from build123d import *

# Parameters (mm, degrees)
SKETCH1_R           = 3.1877
BOSS_EXTRUDE1_DEPTH = 9.525


with BuildPart() as part:
    # Sketch1 → Boss-Extrude1 (new body)
    with BuildSketch(Plane.XY):
        with BuildLine():
            Line((-19.84375, -1.016), (-18.881836189, -1.016))
            ThreePointArc((-18.881836189, -1.016), (-13.4874, 1.4478), (-8.092963811, -1.016))
            Line((-8.092963811, -1.016), (12.583078625, -6.944759764))
            ThreePointArc((12.583078625, -6.944759764), (19.827318682, -1.116916975), (13.49375, 5.6896))
            Line((13.49375, 5.6896), (-13.49375, 5.6896))
            ThreePointArc((-13.49375, 5.6896), (-17.983878061, 3.829728061), (-19.84375, -0.6604))
            Line((-19.84375, -0.6604), (-19.84375, -1.016))
        make_face()
        with Locations((13.49375, -0.6604)):
            Circle(SKETCH1_R, mode=Mode.SUBTRACT)
    extrude(amount=-BOSS_EXTRUDE1_DEPTH)


solid = part.part
The listing builds one solid part. Answer for the finished solid, in the listing's coordinates (mm). A direction names the side the tool comes from. Give positions to 0.01 mm unless a question says otherwise; leave off trailing zeros. Order: outer loops, then holes, each group sorted by start corner. A loop starts at its lowest first (then second) coordinate and runs counter-clockwise, first axis right, second up. Notation, with made-up numbers: (9, 71.25) - (21, 71.25) arc R12 cw to (21, 90.25) - close; hole circle Ø10 at (-38.5, 34). An arc over 180 degrees is marked (long way). Use one line per item in the form item = value.
1) Find section B-B on z = -7.75. Determine the outline of the cut face in (x, y), and give its area (3 significant figures).
Verdict:
outline = (-19.84, -1.02) - (-18.88, -1.02) arc R7.14 cw to (-8.09, -1.02) - (12.58, -6.94) arc R6.35 ccw (long way) to (13.49, 5.69) - (-13.49, 5.69) arc R6.35 ccw to (-19.84, -0.66) - close; hole circle Ø6.38 at (13.49, -0.66)
area = 295 mm^2
2) Find section C-C on x = 15.5. Determine the outline of the cut face in (y, z) (3 decimals).
Verdict:
outline = (-6.685, -9.525) - (-3.138, -9.525) - (-3.138, 0) - (-6.685, 0) - close; (1.817, -9.525) - (5.364, -9.525) - (5.364, 0) - (1.817, 0) - close
3) Each of these flat-tipped pins is pushed along its axis until it touches: pin 1 (1.5 mm diameter, centred on x = -1, z = -3, fed in from -Y); pin 2 (1 mm diameter, centred on x = -14.5, z = -8, fed in from -Y). Where does it stop, or does it pass through?
Verdict:
pin_1 = -3.26
pin_2 = 1.29
4) The mould has two halves that part along X. Classify faces 3 (the cylindrical face through (16.44, -1.88, -4.7)), 4 (the flat face through (4, 1, 0)), 5 (the cylindrical face through (-13.573, 1.447, -4.696)), 6 (the cylindrical face through (-17.934, 3.879, -4.696)): released by +X, released by -X, zero draft, split by the parting line, or undercut.
Verdict:
face_3 = undercut
face_4 = zero draft
face_5 = undercut
face_6 = released by -X
5) Find section D-D on y = 2. Determine the outline of the cut face in (x, z) (3 decimals).
Verdict:
outline = (-19.26, -9.525) - (11.738, -9.525) - (11.738, 0) - (-19.26, 0) - close; (15.25, -9.525) - (19.26, -9.525) - (19.26, 0) - (15.25, 0) - close
6) Find section A-A on y = 0. Determine the outline of the cut face in (x, z) (3 decimals).
Verdict:
outline = (-19.809, -9.525) - (-17.797, -9.525) - (-17.797, 0) - (-19.809, 0) - close; (-9.178, -9.525) - (10.375, -9.525) - (10.375, 0) - (-9.178, 0) - close; (16.612, -9.525) - (19.809, -9.525) - (19.809, 0) - (16.612, 0) - close
7) Consider probe 1 along Y at (x, z) = (14.5, -3.5); probe 2 along X at (y, z) = (2, -0.25); probe 3 along Y at (x, z) = (11, -6.5). Determine where each line is inside the solid, lowest interval first. Write a range as [from, to].
Verdict:
probe_1 = [-6.93, -3.69], [2.36, 5.61]
probe_2 = [-19.26, 11.74], [15.25, 19.26]
probe_3 = [-6.49, -2.65], [1.33, 5.69]
8) For faces 1 (the flat face through (-19.4, -1.016, -4.7)), 2 (the flat face through (0, 5.69, -5)), determine the directions among +Z, -Z, +X, -X, +Y, -Y from which every point of the face is accessible in a straight line to the end or side of a thin tool.
Verdict:
face_1 = +Z, -Z, -X, -Y
face_2 = +Z, -Z, +X, -X, +Y
